Geometry check sheet. Reference: the model listing, model coordinates, mm. Round coordinates to 2 decimals unless told otherwise and drop trailing zeros. Order: outer loops, then holes, each group sorted by start corner. A loop starts at its lowest first (then second) coordinate and runs counter-clockwise, first axis right, second up.
(1) Go/stop test with a flat-tipped pin: pin 1 (1.9 mm diameter, centred on y = -1.5, z = 57, fed in from -X). Record where the tip stops, or that it passes through.
(2) Sectioned sample at B-B (z = 50.8). Give the number of separate pieces and of enclosed holes in the cut face, plus the area to 3 significant figures.
(3) Sectioned sample at A-A (x = 571.5). Record the boundary of the cut face in (y, z).
(4) Material ranges on line 1 along X through (y, z) = (-1.5, 26); line 2 along Z through (x, y) = (698.5, -2); line 3 along Z through (x, y) = (133.5, -1), recorded low to high.
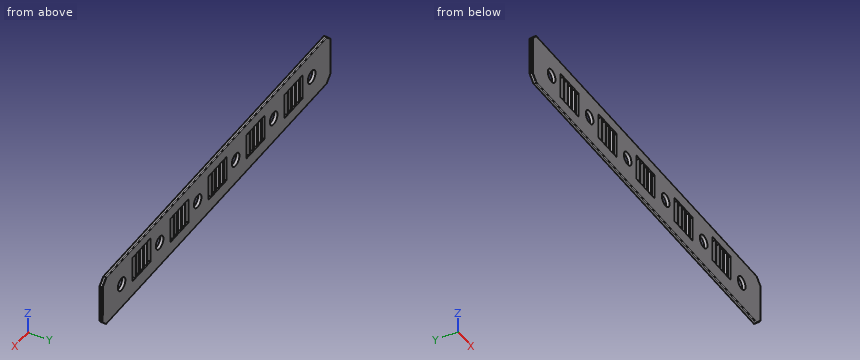
from build123d import *

# Parameters (mm, degrees)
F0_W     = 762
F0_H     = 101.6
F0_R     = 12.7
F1_DEPTH = 6.35
F2_W     = 9.525
F2_H     = 50.8
F3_DEPTH = 6.351
F4_SIZE  = 12.7
F5_R     = 1.6002


with BuildPart() as f1:
    # F0 (on Front) → F1 (new body)
    with BuildSketch(Plane.XZ):
        with Locations((381, 50.8)):
            Rectangle(F0_W, F0_H)
        with Locations((63.5, 50.8)):
            Circle(F0_R, mode=Mode.SUBTRACT)
        with Locations((190.5, 50.8)):
            Circle(F0_R, mode=Mode.SUBTRACT)
        with Locations((317.5, 50.8)):
            Circle(F0_R, mode=Mode.SUBTRACT)
        with Locations((444.5, 50.8)):
            Circle(F0_R, mode=Mode.SUBTRACT)
        with Locations((571.5, 50.8)):
            Circle(F0_R, mode=Mode.SUBTRACT)
        with Locations((698.5, 50.8)):
            Circle(F0_R, mode=Mode.SUBTRACT)
    extrude(amount=F1_DEPTH)

    # F2 (on face) → F3 (cut, through all)
    with BuildSketch(Plane.XZ.offset(6.35)):
        with Locations((98.4377, 50.8)):
            Rectangle(F2_W, F2_H)
        with Locations((111.1377, 50.8)):
            Rectangle(F2_W, F2_H)
        with Locations((123.8377, 50.8)):
            Rectangle(F2_W, F2_H)
        with Locations((136.5377, 50.8)):
            Rectangle(F2_W, F2_H)
        with Locations((149.2377, 50.8)):
            Rectangle(F2_W, F2_H)
        with Locations((225.4377, 53.3135051852)):
            Rectangle(F2_W, F2_H)
        with Locations((238.1377, 53.3135051852)):
            Rectangle(F2_W, F2_H)
        with Locations((250.8377, 53.3135051852)):
            Rectangle(F2_W, F2_H)
        with Locations((263.5377, 53.3135051852)):
            Rectangle(F2_W, F2_H)
        with Locations((276.2377, 53.3135051852)):
            Rectangle(F2_W, F2_H)
        with Locations((352.4377, 53.2665329998)):
            Rectangle(F2_W, F2_H)
        with Locations((365.1377, 53.2665329998)):
            Rectangle(F2_W, F2_H)
        with Locations((377.8377, 53.2665329998)):
            Rectangle(F2_W, F2_H)
        with Locations((390.5377, 53.2665329998)):
            Rectangle(F2_W, F2_H)
        with Locations((403.2377, 53.2665329998)):
            Rectangle(F2_W, F2_H)
        with Locations((479.4377, 51.6235756701)):
            Rectangle(F2_W, F2_H)
        with Locations((492.1377, 51.6235756701)):
            Rectangle(F2_W, F2_H)
        with Locations((504.8377, 51.6235756701)):
            Rectangle(F2_W, F2_H)
        with Locations((517.5377, 51.6235756701)):
            Rectangle(F2_W, F2_H)
        with Locations((530.2377, 51.6235756701)):
            Rectangle(F2_W, F2_H)
        with Locations((606.4377, 56.4514326876)):
            Rectangle(F2_W, F2_H)
        with Locations((619.1377, 56.4514326876)):
            Rectangle(F2_W, F2_H)
        with Locations((631.8377, 56.4514326876)):
            Rectangle(F2_W, F2_H)
        with Locations((644.5377, 56.4514326876)):
            Rectangle(F2_W, F2_H)
        with Locations((657.2377, 56.4514326876)):
            Rectangle(F2_W, F2_H)
    extrude(amount=-F3_DEPTH, mode=Mode.SUBTRACT)

    # F4
    f4_edges = [f1.edges().sort_by_distance(p)[0] for p in [
        (0, -3.175, 101.6),
        (0, -3.175, 0),
        (762, -3.175, 0),
        (762, -3.175, 101.6),
    ]]
    chamfer(f4_edges, length=F4_SIZE)

    # F5
    f5_edges = [f1.edges().sort_by_distance(p)[0] for p in [
        (381, -6.35, 101.6),
        (381, 0, 101.6),
        (6.35, -6.35, 95.25),
        (6.35, 0, 95.25),
        (0, -6.35, 50.8),
        (0, 0, 50.8),
        (6.35, -6.35, 6.35),
        (6.35, 0, 6.35),
        (381, -6.35, 0),
        (381, 0, 0),
        (755.65, -6.35, 95.25),
        (755.65, 0, 95.25),
        (762, 0, 50.8),
        (762, -6.35, 50.8),
        (755.65, -6.35, 6.35),
    ]]
    fillet(f5_edges, radius=F5_R)


solid = f1.part
Answer below:
1. pin 1: stops at x = 0
2. separate pieces: 32
2. enclosed holes: 0
2. area: 2,360 mm2
3. outline: (-6.35, 1.6) arc R1.6 ccw to (-4.75, 0) - (-1.6, 0) arc R1.6 ccw to (0, 1.6) - (0, 38.1) - (-6.35, 38.1) - close; (-6.35, 63.5) - (0, 63.5) - (0, 100) arc R1.6 ccw to (-1.6, 101.6) - (-4.75, 101.6) arc R1.6 ccw to (-6.35, 100) - close
4. line 1: x = 0 to 93.68, 103.2 to 106.38, 115.9 to 119.08, 128.6 to 131.78, 141.3 to 144.48, 154 to 762
4. line 2: z = 0 to 38.1, 63.5 to 101.6
4. line 3: z = 0.12 to 25.4, 76.2 to 101.48
